from build123d import *

# Parameters (mm, degrees)
SKETCH1_W    = 187
SKETCH1_H    = 112
SKETCH1_R    = 1.425
SKETCH1_W_2  = 163
SKETCH1_H_2  = 88
BASE_DEPTH   = 3
SKETCH3_W    = 187
SKETCH3_H    = 112
SKETCH3_R    = 1.425
SKETCH3_W_2  = 176.5
SKETCH3_H_2  = 101.5
EDGE_2_DEPTH = 10
FILLET1_R    = 1


with BuildPart() as part:
    # Sketch1 → Base (new body)
    with BuildSketch(Plane(origin=(0, 0, 0), x_dir=(1, 0, 0), z_dir=(0, 1, 0))):
        Rectangle(SKETCH1_W, SKETCH1_H)
        with Locations(Location((-89.5, -52, 0), (0, 0, 270))):
            Circle(SKETCH1_R, mode=Mode.SUBTRACT)
        with Locations(Location((89.5, -52, 0), (0, 0, 270))):
            Circle(SKETCH1_R, mode=Mode.SUBTRACT)
        with Locations(Location((89.5, 52, 0), (0, 0, 270))):
            Circle(SKETCH1_R, mode=Mode.SUBTRACT)
        with Locations(Location((-89.5, 52, 0), (0, 0, 270))):
            Circle(SKETCH1_R, mode=Mode.SUBTRACT)
        with Locations(Location((-83.5, -46, 0), (0, 0, 270))):
            Circle(SKETCH1_R, mode=Mode.SUBTRACT)
        with Locations(Location((0, -46, 0), (0, 0, 270))):
            Circle(SKETCH1_R, mode=Mode.SUBTRACT)
        with Locations(Location((83.5, -46, 0), (0, 0, 270))):
            Circle(SKETCH1_R, mode=Mode.SUBTRACT)
        with Locations(Location((0, 46, 0), (0, 0, 270))):
            Circle(SKETCH1_R, mode=Mode.SUBTRACT)
        with Locations(Location((83.5, 46, 0), (0, 0, 270))):
            Circle(SKETCH1_R, mode=Mode.SUBTRACT)
        with Locations(Location((-83.5, 46, 0), (0, 0, 270))):
            Circle(SKETCH1_R, mode=Mode.SUBTRACT)
        Rectangle(SKETCH1_W_2, SKETCH1_H_2, mode=Mode.SUBTRACT)
    extrude(amount=BASE_DEPTH)

    # Sketch3 → Edge 2 (add)
    with BuildSketch(Plane(origin=(0, 3, 0), x_dir=(1, 0, 0), z_dir=(0, 1, 0))):
        Rectangle(SKETCH3_W, SKETCH3_H)
        with Locations(Location((-89.5, -52, 0), (0, 0, 270))):
            Circle(SKETCH3_R, mode=Mode.SUBTRACT)
        with Locations(Location((89.5, -52, 0), (0, 0, 270))):
            Circle(SKETCH3_R, mode=Mode.SUBTRACT)
        with Locations(Location((89.5, 52, 0), (0, 0, 270))):
            Circle(SKETCH3_R, mode=Mode.SUBTRACT)
        with Locations(Location((-89.5, 52, 0), (0, 0, 270))):
            Circle(SKETCH3_R, mode=Mode.SUBTRACT)
        Rectangle(SKETCH3_W_2, SKETCH3_H_2, mode=Mode.SUBTRACT)
    extrude(amount=EDGE_2_DEPTH)

    # Fillet1
    fillet1_edges = [part.edges().sort_by_distance(p)[0] for p in [
        (0, 0, -56),
        (93.5, 0, 0),
        (0, 0, 56),
        (-93.5, 0, 0),
        (-93.5, 6.5, -56),
        (93.5, 6.5, -56),
        (93.5, 6.5, 56),
        (-93.5, 6.5, 56),
    ]]
    fillet(fillet1_edges, radius=FILLET1_R)


solid = part.part
Design review of the part built by this model. Coordinates are the model's own, in mm. A direction names the side the tool comes from. Coordinates: 2 decimals unless noted, no trailing zeros. Loops run counter-clockwise (first coordinate to the right, second up) from the corner with the lowest first, then second, coordinate; pieces in that order, holes last. Notation, with made-up numbers: (48.25, -21) - (68.25, -21) arc R13 ccw to (68.25, -17) - close; hole circle Ø10 at (73, 74.25). An arc over 180 degrees is marked (long way). Use CSV: the item, a comma, the result in double quotes. Start each with the question number.
1. To check wall thickness, follow probe 1 along X at (y, z) = (5.5, -52) (3 decimals); probe 2 along X at (y, z) = (2.15, -46) (3 decimals); probe 3 along Z at (x, y) = (-83.5, 2.15) (3 decimals). State the ranges of each line that lie inside material, in increasing order.
2. Add section C-C on x = 30. Give the boundary of the cut face in (y, z), plus the area to 3 significant figures.
3. Add section A-A on z = -21. Give the boundary of the cut face in (x, y), plus the area to 3 significant figures.
4. For faces 1 (the flat face through (-1, 8, 50.75)), 2 (the flat face through (6, 0, 45)), list the 3-axis set-ups (+Z, -Z, +X, -X, +Y, -Y) from which the entire face can be reached by the end or side of a thin tool; tool diameter is ignored.
5. Clearance check with flat-ended pins moving along their axes: pin 1 (8 mm diameter, centred on x = -9.5, z = 41.5, fed in from -Y); pin 2 (1.7 mm diameter, centred on x = 0, z = 46, fed in from +Y); pin 3 (10 mm diameter, centred on x = -54, z = -43, fed in from +Y). State where each tip first meets the part, or that it passes through.
6. Mouldability with a two-part tool opening along Z and no side actions: class faces 3 (the flat face through (-1, 8, -50.75)), 4 (the flat face through (-1, 7, -56)), 5 (the flat face through (6, 3, -45)), 6 (the flat face through (-1, 7, 56)) as released by +Z, released by -Z, zero draft, split by the parting line, or undercut.
7. Add section B-B on y = 8.5. Give the boundary of the cut face in (x, z) (3 decimals), plus the area to 3 significant figures.
Resolved:
1,probe 1,"-93.5 to -90.925, -88.075 to 88.075, 90.925 to 93.5"
1,probe 2,"-93.5 to -84.925, -82.075 to -1.425, 1.425 to 82.075, 84.925 to 93.5"
1,probe 3,"-56 to -47.425, -44.575 to 44.575, 47.425 to 56"
2,outline,"(0, -55) arc R1 ccw to (1, -56) - (13, -56) - (13, -50.75) - (3, -50.75) - (3, -44) - (0, -44) - close; (0, 44) - (3, 44) - (3, 50.75) - (13, 50.75) - (13, 56) - (1, 56) arc R1 ccw to (0, 55) - close"
2,area,"177 mm2"
3,outline,"(-93.5, 1) arc R1 ccw to (-92.5, 0) - (-81.5, 0) - (-81.5, 3) - (-88.25, 3) - (-88.25, 13) - (-93.5, 13) - close; (81.5, 0) - (92.5, 0) arc R1 ccw to (93.5, 1) - (93.5, 13) - (88.25, 13) - (88.25, 3) - (81.5, 3) - close"
3,area,"177 mm2"
4,face 1,"+Y"
4,face 2,"+Z, -Z, +X, -X, -Y"
5,pin 1,"y = 0"
5,pin 2,"through"
5,pin 3,"y = 3"
6,face 3,"undercut"
6,face 4,"released by -Z"
6,face 5,"undercut"
6,face 6,"released by +Z"
7,outline,"(-93.5, -55) arc R1 ccw to (-92.5, -56) - (92.5, -56) arc R1 ccw to (93.5, -55) - (93.5, 55) arc R1 ccw to (92.5, 56) - (-92.5, 56) arc R1 ccw to (-93.5, 55) - close; hole circle Ø2.85 at (-89.5, -52); hole circle Ø2.85 at (-89.5, 52); hole (-88.25, -50.75) - (88.25, -50.75) - (88.25, 50.75) - (-88.25, 50.75) - close; hole circle Ø2.85 at (89.5, -52); hole circle Ø2.85 at (89.5, 52)"
7,area,"3,000 mm2"
